The model under review builds one solid part; all positions refer to its coordinate system, in mm. Face numbers are marked on the shaded views. Round coordinates to 2 decimals unless told otherwise and drop trailing zeros. Loops run counter-clockwise (first coordinate to the right, second up) from the corner with the lowest first, then second, coordinate; pieces in that order, holes last. Notation, with made-up numbers: (45.5, 70) -> (59.5, 70) arc R21 cw to (59.5, 108) -> close; hole circle Ø1 at (25.5, 5.5). An arc over 180 degrees is marked (long way). Use a Markdown table: item, result. Add a question column.
1) Consider section D-D on x = 10.5. Give the boundary of the cut face in (y, z), plus the area to 3 significant figures.
2) Mouldability with a two-part tool opening along X and no side actions: class the marked faces 1, 2, 3 and 4 as released by +X, released by -X, zero draft, split by the parting line, or undercut.
3) Wall thickness on probe 1 along X at (y, z) = (13.5, 0.85); probe 2 along X at (y, z) = (15.5, 0.9); probe 3 along Y at (x, z) = (4.25, 0.45): over which ranges is each line inside the solid? List them lowest first.
4) Consider section B-B on z = 0.3. Give the boundary of the cut face in (x, y).
5) Consider section C-C on x = 5. Give the boundary of the cut face in (y, z).
6) Insertion check: pin 1 (2 mm diameter, centred on x = 15, y = 15.5, fed in from +Z). The pin has a flat end and moves straight along its axis. Give the tip position at first contact, or say it passes through.
7) Consider section A-A on y = 15.5. Give the boundary of the cut face in (x, z).
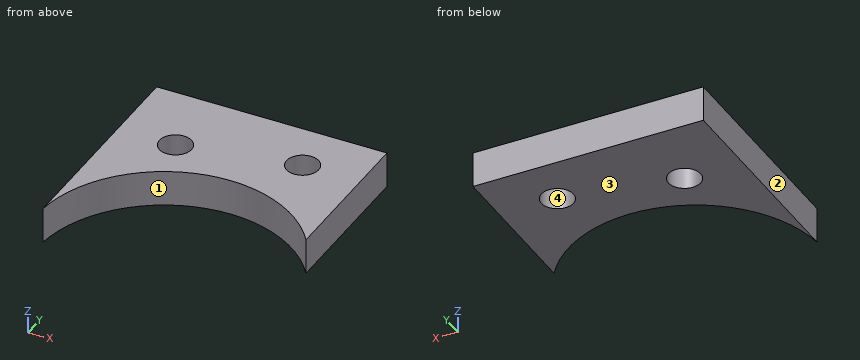
from build123d import *

# Parameters (mm, degrees)
SKETCH1_R           = 1.4
BOSS_EXTRUDE1_DEPTH = 3.1


with BuildPart() as part:
    # Sketch1 → Boss-Extrude1 (new body)
    with BuildSketch(Plane.XY):
        with BuildLine():
            Line((0, 0.939361485), (0, 20))
            Line((0, 20), (20, 20))
            Line((20, 20), (20, 6.425138131))
            ThreePointArc((20, 6.425138131), (8.087067166, 10.656404818), (0, 0.939361485))
        make_face()
        with Locations(Location((5, 13.5, 0), (0, 0, 180))):
            Circle(SKETCH1_R, mode=Mode.SUBTRACT)
        with Locations(Location((15, 15.5, 0), (0, 0, 180))):
            Circle(SKETCH1_R, mode=Mode.SUBTRACT)
    extrude(amount=BOSS_EXTRUDE1_DEPTH)


solid = part.part
Result set:
| question | item | result |
|---|---|---|
| 1 | outline | (11.04, 0) -> (20, 0) -> (20, 3.1) -> (11.04, 3.1) -> close |
| 1 | area | 27.8 mm2 |
| 2 | face 1 | undercut |
| 2 | face 2 | released by -X |
| 2 | face 3 | zero draft |
| 2 | face 4 | undercut |
| 3 | probe 1 | 0 to 3.6, 6.4 to 20 |
| 3 | probe 2 | 0 to 13.6, 16.4 to 20 |
| 3 | probe 3 | 8.74 to 12.32, 14.68 to 20 |
| 4 | outline | (0, 0.94) arc R11.05 cw to (20, 6.43) -> (20, 20) -> (0, 20) -> close; hole circle Ø2.8 at (5, 13.5); hole circle Ø2.8 at (15, 15.5) |
| 5 | outline | (9.27, 0) -> (12.1, 0) -> (12.1, 3.1) -> (9.27, 3.1) -> close; (14.9, 0) -> (20, 0) -> (20, 3.1) -> (14.9, 3.1) -> close |
| 6 | pin 1 | through |
| 7 | outline | (0, 0) -> (13.6, 0) -> (13.6, 3.1) -> (0, 3.1) -> close; (16.4, 0) -> (20, 0) -> (20, 3.1) -> (16.4, 3.1) -> close |
